Source: CAD feature listing. Evaluate the final solid. Frame: model axes, mm. A direction names the side the tool comes from. Give positions to 0.01 mm unless a question says otherwise; leave off trailing zeros. Loops run counter-clockwise (first coordinate to the right, second up) from the corner with the lowest first, then second, coordinate; pieces in that order, holes last.
Solid Edge part; units mm, degrees
sketch "Sketch1" plane through (0, 0, 0) normal (0, 0, 1) x (1, 0, 0)
  circle A0 centre (-48.678, 43.9628) radius 40
extrude "Protrusion1" add sketch "Sketch1" along normal blind 100
sketch "Sketch2" plane through (0, 0, 0) normal (0, 0, 1) x (1, 0, 0)
  circle A0 centre (-48.678, 43.9628) radius 15
extrude "ExtrudedProtrusion_3" add sketch "Sketch2" against normal blind 10
sketch "Sketch3" plane through (-48.678, 43.9628, -10) normal (0, 0, -1) x (0, -1, 0)
  circle A0 centre (0, 0) radius 5
extrude "ExtrudedProtrusion_4" add sketch "Sketch3" along normal blind 10
(1) Ray query, line 1 along Z through (x, y) = (-48, 27); line 2 along X through (y, z) = (42.5, 34); line 3 along Z through (x, y) = (-36.5, 45.5). Return the intervals inside material, ascending.
A:
line 1: z = 0 to 100
line 2: x = -88.65 to -8.7
line 3: z = -10 to 100
(2) Section C-C, the plane z = 89. Return the cut outline in (x, y), then the cut area to 3 significant figures.
A:
outline: circle Ø80 at (-48.68, 43.96)
area: 5,030 mm2
(3) Section D-D, the plane x = -71. Return the cut outline in (y, z).
A:
outline: (10.77, 0) - (77.16, 0) - (77.16, 100) - (10.77, 100) - close
(4) First-contact query: pin 1 (6 mm diameter, centred on y = 49.5, z = 0, fed in from +X); pin 2 (4 mm diameter, centred on y = 19.5, z = 62, fed in from -X); pin 3 (5 mm diameter, centred on y = 18, z = 57.5, fed in from -X). Flat tips, straight axial feed; report the tip coordinate or a pass-through.
A:
pin 1: stops at x = -8.76
pin 2: stops at x = -81.78
pin 3: stops at x = -81.07
(5) Section A-A, the plane x = -55.5. Return the cut outline in (y, z).
A:
outline: (4.55, 0) - (30.6, 0) - (30.6, -10) - (57.32, -10) - (57.32, 0) - (83.38, 0) - (83.38, 100) - (4.55, 100) - close
(6) Reachability of faces 1 (the cylindrical face through (-53.114, 41.656, -14.93)), 2 (the cylindrical face through (-88.64, 42.2, 49.3)) from +Z, -Z, +X, -X, +Y, -Y: full face, straight path, thin tool, end or side. Return the list, or none.
A:
face 1: -Z
face 2: +Z, -Z
(7) Section B-B, the plane y = 36.5. Return the cut outline in (x, z).
A:
outline: (-87.98, 0) - (-61.69, 0) - (-61.69, -10) - (-35.67, -10) - (-35.67, 0) - (-9.38, 0) - (-9.38, 100) - (-87.98, 100) - close
